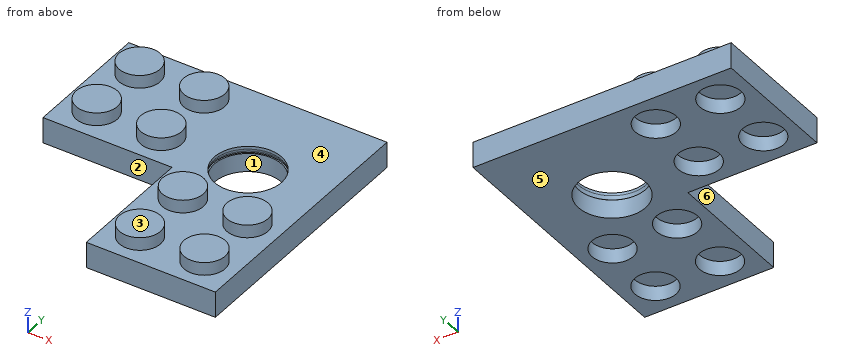
from build123d import *

# Parameters (mm, degrees)
SKETCH1_R           = 4.15
BOSS_EXTRUDE1_DEPTH = 3.2
CUT_EXTRUDE3_START  = 3.2
SKETCH1_3_R         = 2.55
CUT_EXTRUDE3_DEPTH  = 1.8
SKETCH1_4_R         = 2.55
BOSS_EXTRUDE2_DEPTH = 1.6


with BuildPart() as part:
    # Sketch1 → Boss-Extrude1 (new body)
    with BuildSketch(Plane(origin=(0, 0, -17.400004116), x_dir=(-1, 0, 0), z_dir=(0, 0, -1))):
        Polygon((2.501166814, -72.5), (-13.498833186, -72.5), (-13.498833186, -40.5), (18.501166814, -40.5), (18.501166814, -56.5), (2.501166814, -56.5), align=None)
        with Locations(Location((-4.246216621, -52.5, 0), (0, 0, 90))):
            Circle(SKETCH1_R, mode=Mode.SUBTRACT)
    extrude(amount=BOSS_EXTRUDE1_DEPTH)

    # Sketch1<3> → Cut-Extrude3 (cut)
    with BuildSketch(Plane(origin=(0, 0, -17.400004116), x_dir=(-1, 0, 0), z_dir=(0, 0, -1)).offset(CUT_EXTRUDE3_START)):
        with Locations(Location((6.501166814, -52.5, 0), (0, 0, 180))):
            Circle(SKETCH1_3_R)
        with Locations(Location((6.501166814, -44.5, 0), (0, 0, 180))):
            Circle(SKETCH1_3_R)
        with Locations(Location((14.501166814, -44.5, 0), (0, 0, 180))):
            Circle(SKETCH1_3_R)
        with Locations(Location((14.501166814, -52.5, 0), (0, 0, 180))):
            Circle(SKETCH1_3_R)
        with Locations(Location((-9.498833186, -60.5, 0), (0, 0, 180))):
            Circle(SKETCH1_3_R)
        with Locations(Location((-1.498833186, -60.5, 0), (0, 0, 180))):
            Circle(SKETCH1_3_R)
        with Locations(Location((-1.498833186, -68.5, 0), (0, 0, 180))):
            Circle(SKETCH1_3_R)
        with Locations(Location((-9.498833186, -68.5, 0), (0, 0, 180))):
            Circle(SKETCH1_3_R)
    extrude(amount=-CUT_EXTRUDE3_DEPTH, mode=Mode.SUBTRACT)

    # Sketch1<4> → Boss-Extrude2 (add)
    with BuildSketch(Plane(origin=(0, 0, -17.400004116), x_dir=(-1, 0, 0), z_dir=(0, 0, -1))):
        with Locations(Location((6.501166814, -44.5, 0), (0, 0, 180))):
            Circle(SKETCH1_4_R)
        with Locations(Location((14.501166814, -44.5, 0), (0, 0, 180))):
            Circle(SKETCH1_4_R)
        with Locations(Location((14.501166814, -52.5, 0), (0, 0, 180))):
            Circle(SKETCH1_4_R)
        with Locations(Location((6.501166814, -52.5, 0), (0, 0, 180))):
            Circle(SKETCH1_4_R)
        with Locations(Location((-1.498833186, -60.5, 0), (0, 0, 180))):
            Circle(SKETCH1_4_R)
        with Locations(Location((-1.498833186, -68.5, 0), (0, 0, 180))):
            Circle(SKETCH1_4_R)
        with Locations(Location((-9.498833186, -60.5, 0), (0, 0, 180))):
            Circle(SKETCH1_4_R)
        with Locations(Location((-9.498833186, -68.5, 0), (0, 0, 180))):
            Circle(SKETCH1_4_R)
    extrude(amount=-BOSS_EXTRUDE2_DEPTH)

    # Sketch2 → Cut-Revolve1 (revolve, cut)
    with BuildSketch(Plane(origin=(4.246216621, -52.5, -15.300004116), x_dir=(0, 0, 1), z_dir=(-1, 0, 0))):
        Polygon((-2.846789772, 4.335), (-1.913929092, 3.899999921), (-3, 3.900000008), (-3, 4.335), align=None)
    revolve(axis=Axis((4.246216621, -52.5, -17.665004136), (0, 0, 1)), mode=Mode.SUBTRACT)


solid = part.part
Geometry: final body of the model. Coordinates: model frame, mm. Face numbers are marked on the shaded views. A direction names the side the tool comes from. Give positions to 0.01 mm unless a question says otherwise; leave off trailing zeros. Order: outer loops, then holes, each group sorted by start corner. A loop starts at its lowest first (then second) coordinate and runs counter-clockwise, first axis right, second up. Notation, with made-up numbers: (-1.5, 75) -> (4.5, 75) arc R9 ccw to (4.5, 83) -> close; hole circle Ø1 at (-19.5, 75.5). An arc over 180 degrees is marked (long way). Write each question's results on one line, items separated by ' | '.
1) Cut plane B-B (z = -19.5). Give the number of separate pieces and of enclosed holes in the cut face, and give its area (3 significant figures).
Geometry says:
separate pieces: 1 | enclosed holes: 9 | area: 550 mm²
2) Set-up query: the marked faces 5 and 6. Return all of +Z, -Z, +X, -X, +Y, -Y with unobstructed straight access to the full face (end or side cutting, diameter ignored); none if empty.
Geometry says:
face 5: -Z, +X, -X, +Y, -Y | face 6: +Z, -Z, -X, -Y
3) Line query: line 1 along X through (y, z) = (-44.5, -19.7); line 2 along X through (y, z) = (-52.5, -18.15); line 3 along X through (y, z) = (-43.5, -20.1). Output: solid intervals per line, ascending.
Geometry says:
line 1: x = -18.5 to -17.05, -11.95 to -9.05, -3.95 to 13.5 | line 2: x = -18.5 to -0.09, 8.58 to 13.5 | line 3: x = -18.5 to -16.85, -12.16 to -8.85, -4.16 to 13.5
4) Cut plane D-D (y = -68.5). Output: boundary loops of the cut face in (x, z).
Geometry says:
outline: (-2.5, -20.6) -> (-1.05, -20.6) -> (-1.05, -18.8) -> (4.05, -18.8) -> (4.05, -20.6) -> (6.95, -20.6) -> (6.95, -18.8) -> (12.05, -18.8) -> (12.05, -20.6) -> (13.5, -20.6) -> (13.5, -17.4) -> (12.05, -17.4) -> (12.05, -15.8) -> (6.95, -15.8) -> (6.95, -17.4) -> (4.05, -17.4) -> (4.05, -15.8) -> (-1.05, -15.8) -> (-1.05, -17.4) -> (-2.5, -17.4) -> close
5) Cut plane C-C (x = 11). Output: boundary loops of the cut face in (y, z).
Geometry says:
outline: (-72.5, -20.6) -> (-70.56, -20.6) -> (-70.56, -18.8) -> (-66.44, -18.8) -> (-66.44, -20.6) -> (-62.56, -20.6) -> (-62.56, -18.8) -> (-58.44, -18.8) -> (-58.44, -20.6) -> (-40.5, -20.6) -> (-40.5, -17.4) -> (-58.44, -17.4) -> (-58.44, -15.8) -> (-62.56, -15.8) -> (-62.56, -17.4) -> (-66.44, -17.4) -> (-66.44, -15.8) -> (-70.56, -15.8) -> (-70.56, -17.4) -> (-72.5, -17.4) -> close
6) Draft query along Y for the marked faces 1, 2, 3 and 4. Return one class per face: released by +Y, released by -Y, zero draft, split by the parting line, or undercut.
Geometry says:
face 1: undercut | face 2: released by -Y | face 3: zero draft | face 4: undercut
7) First-contact query: pin 1 Ø10 at (x, y) = (2.5, -52) entering from -Z; pin 2 Ø3 at (x, y) = (9.5, -60.5) entering from -Z; pin 3 Ø5 at (x, y) = (4.25, -52.5) entering from -Z; pin 4 Ø1.5 at (x, z) = (-7.5, -17.5) entering from -Y. Flat tips, straight axial feed; report the tip coordinate or a pass-through.
Geometry says:
pin 1: stops at z = -20.6 | pin 2: stops at z = -18.8 | pin 3: passes through | pin 4: stops at y = -56.5
